Part model, mm, in its own coordinate system. A direction names the side the tool comes from. Coordinates: 2 decimals unless noted, no trailing zeros. Order: outer loops, then holes, each group sorted by start corner. A loop starts at its lowest first (then second) coordinate and runs counter-clockwise, first axis right, second up.
1) Cut at D-D (y = 27.5). List the corners of the cut face in (x, z), and give its area (3 significant figures).
2) Cut at C-C (x = -14). List the corners of the cut face in (y, z), and give its area (3 significant figures).
3) Pin check, flat tips, straight feed: pin 1 Ø0.9 at (x, y) = (-23.5, 33) entering from +Z; pin 2 Ø12 at (x, y) = (-24, -6.5) entering from -Z; pin 3 Ø1.2 at (x, z) = (-30.7, 5) entering from -Y; pin 4 Ø6 at (x, y) = (-41.5, 27) entering from +Z. Stop position of each tip, or through.
4) Cut at B-B (y = 2.5). List the corners of the cut face in (x, z), and give its area (3 significant figures).
5) Tool access for faces 1 (the cylindrical face through (-11.004, 31.9, 4.958)), 2 (the cylindrical face through (-31.7, -14.1, 5.1)), 3 (the flat face through (-18, 10.185, 1)), 4 (the flat face through (-10.704, 10, 5)): list every direction of +Z, -Z, +X, -X, +Y, -Y with a clear straight run to the whole face (end or side of a thin tool).
6) Wall check: L1, parallel to X at y = 32.5, z = 5; L2, parallel to Y at x = -36, z = 7; L3, parallel to Y at x = -33, z = 1.5. Give the ranges that are in metal, low to high.
7) Mould opens along Z. For faces 5 (the cylindrical face through (-43.7, -14.1, 5.1)), 6 (the flat face through (-28, -15, 8)), 7 (the cylindrical face through (-11.004, -13.53, 5.042)) say: +Z half, -Z half, draft (parallel to the pull), parting line (faces both ways), or undercut.
8) Cut at A-A (z = 5). Give the number of separate pieces and of enclosed holes in the cut face, and give its area (3 significant figures).
Autodesk Inventor part; units mm, degrees
ref_plane "YZ Plane" through (0, 0, 0) normal (1, 0, 0) x (0, 1, 0)
ref_plane "XZ Plane" through (0, 0, 0) normal (0, 1, 0) x (-1, 0, 0)
ref_plane "XY Plane" through (0, 0, 0) normal (0, 0, 1) x (1, 0, 0)
sketch "Sketch1" plane through (0, 0, 0) normal (0, 0, 1) x (1, 0, 0)
  line L0 (-45.7037, 34.1852) -> (-8.7037, 34.1852)
  line L1 (-8.7037, 34.1852) -> (-8.7037, -15.8148)
  line L2 (-8.7037, -15.8148) -> (-45.7037, -15.8148)
  line L3 (-45.7037, -15.8148) -> (-45.7037, 34.1852)
  line L4 (-43.7037, 32.1852) -> (-10.7037, 32.1852)
  line L5 (-10.7037, 32.1852) -> (-10.7037, -13.8148)
  line L6 (-10.7037, -13.8148) -> (-43.7037, -13.8148)
  line L7 (-43.7037, -13.8148) -> (-43.7037, 32.1852)
  point P0 (0, 0)
  dimension "d0" = 2
  dimension "d1" = 2
  dimension "d2" = 2
  dimension "d3" = 2
  dimension "d4" = 37
  dimension "d5" = 50
extrude "Extrusion1" add sketch "Sketch1" along normal blind 2
sketch "Sketch2" plane through (0, 0, 2) normal (0, 0, 1) x (1, 0, 0)
  line L0 (-43.7037, 32.1852) -> (-10.7037, 32.1852)
  line L1 (-10.7037, -13.8148) -> (-43.7037, -13.8148)
  line L2 (-43.7037, 32.1852) -> (-10.7037, -13.8148) construction
  line L3 (-44.5162, 31.6023) -> (-11.5162, -14.3977)
  line L4 (-9.8912, -13.2319) -> (-42.8912, 32.7681)
  arc A0 (-42.8912, 32.7681) -> (-44.5162, 31.6023) centre (-43.7037, 32.1852) ccw
  arc A1 (-11.5162, -14.3977) -> (-9.8912, -13.2319) centre (-10.7037, -13.8148) ccw
  line L5 (-10.7037, 32.1852) -> (-10.7037, -13.8148)
  line L6 (-10.7037, 32.1852) -> (-43.7037, -13.8148) construction
  line L7 (-11.5162, 32.7681) -> (-44.5162, -13.2319)
  line L8 (-42.8912, -14.3977) -> (-9.8912, 31.6023)
  arc A2 (-9.8912, 31.6023) -> (-11.5162, 32.7681) centre (-10.7037, 32.1852) ccw
  arc A3 (-44.5162, -13.2319) -> (-42.8912, -14.3977) centre (-43.7037, -13.8148) ccw
  point P0 (0, 0)
  point P1 (-27.2037, 9.1852)
  point P2 (-27.2037, 9.1852)
  point P3 (-25.973, 9.1852)
  point P4 (-27.2037, 10.9007)
  point P5 (-28.4344, 9.1852)
  point P6 (-27.2037, 7.4696)
  dimension "d8" = 2
  dimension "d9" = 2
extrude "Extrusion2" add sketch "Sketch2" against normal blind 2 contours L4 L7 L3 A0 | L7 A2 L8 L5 L0 | L0 L5 L8 L4 L7 | L4 L8 L3 L7 | L4 L5 L1 L3 L8 | L3 L8 A3 L7 | L4 A1 L3 L1 L5
sketch "Sketch3" plane through (0, 0, 2) normal (0, 0, 1) x (1, 0, 0)
  line L0 (-45.7037, 34.1852) -> (-45.7037, -15.8148)
  line L1 (-8.7037, -15.8148) -> (-8.7037, 34.1852)
  line L2 (-45.7037, 34.1852) -> (-8.7037, 34.1852)
  line L3 (-8.7037, 34.1852) -> (-8.7037, 32.1852)
  line L4 (-8.7037, 32.1852) -> (-45.7037, 32.1852)
  line L5 (-45.7037, 32.1852) -> (-45.7037, 34.1852)
  line L6 (-45.7037, -15.8148) -> (-8.7037, -15.8148)
  line L7 (-8.7037, -15.8148) -> (-8.7037, -13.8148)
  line L8 (-8.7037, -13.8148) -> (-45.7037, -13.8148)
  line L9 (-45.7037, -13.8148) -> (-45.7037, -15.8148)
  line L10 (-42.473, 32.1852) -> (-11.9344, 32.1852)
  line L11 (-11.9344, -13.8148) -> (-42.473, -13.8148)
  line L12 (-45.7037, -15.8148) -> (-8.7037, -15.8148)
  point P0 (0, 0)
  point P1 (-8.7037, 34.1852)
extrude "Extrusion3" add sketch "Sketch3" along normal blind 6 contours L2 L1 L4 L0 | L8 L1 L6 L0
sketch "Sketch4" plane through (-45.7037, 34.1852, 0) normal (0, 1, 0) x (1, 0, 0)
  line L0 (37, -8) -> (0, -8)
  line L1 (0, 0) -> (0, -8)
  point P0 (45.7037, 0)
  point P1 (3, -5)
  point P2 (15, -5)
  dimension "d14" = 3
  dimension "d15" = 3
  dimension "d16" = 3
  dimension "d17" = 12
hole "Hole1" at (-42.7037, 34.1852, 5) at (-30.7037, 34.1852, 5) direction (0, -1, 0) diameter 2 depth 10 tip angle 118 countersink diameter 5 countersink angle 90
sketch "Sketch5" plane through (-45.7037, -15.8148, 0) normal (0, -1, 0) x (1, 0, 0)
  circle A0 centre (15, 5) radius 1
  circle A1 centre (3, 5) radius 1
  point P0 (45.7037, 0)
hole "Hole2" at (-30.7037, -15.8148, 5) at (-42.7037, -15.8148, 5) direction (0, 1, 0) diameter 2 depth 10 tip angle 118 countersink diameter 5 countersink angle 90
sketch "Sketch6" plane through (0, 0, 0) normal (0, 0, -1) x (-1, 0, 0)
  line L0 (11.9344, -13.8148) -> (42.473, -13.8148)
  line L1 (43.7037, -12.0993) -> (43.7037, 30.4696)
  line L2 (17.7037, -13.8148) -> (43.7037, -13.8148)
  line L3 (43.7037, -13.8148) -> (43.7037, -6.8148)
  line L4 (43.7037, -6.8148) -> (17.7037, -6.8148)
  line L5 (17.7037, -6.8148) -> (17.7037, -13.8148)
  line L6 (17.7037, 32.1852) -> (43.7037, 32.1852)
  line L7 (43.7037, 32.1852) -> (43.7037, 25.1852)
  line L8 (43.7037, 25.1852) -> (17.7037, 25.1852)
  line L9 (17.7037, 25.1852) -> (17.7037, 32.1852)
  line L10 (42.473, 32.1852) -> (11.9344, 32.1852)
  line L11 (45.7037, 34.1852) -> (45.7037, -15.8148)
  line L12 (8.7037, 34.1852) -> (45.7037, 34.1852)
  line L13 (45.7037, -15.8148) -> (8.7037, -15.8148)
  point P0 (0, 0)
  dimension "d35" = 28
  dimension "d36" = 28
  dimension "d37" = 9
  dimension "d38" = 9
extrude "Extrusion4" cut sketch "Sketch6" against normal blind 2
sketch "Sketch7" plane through (0, 0, 0) normal (0, 0, -1) x (-1, 0, 0)
  line L0 (39.9127, -6.8148) -> (37.4513, -6.8148)
  line L1 (43.7037, -13.8148) -> (43.7037, 32.1852)
  line L2 (37.4513, -6.8148) -> (43.7037, -6.8148)
  line L3 (43.7037, -6.8148) -> (43.7037, -4.8148)
  line L4 (43.7037, -4.8148) -> (37.4513, -4.8148)
  line L5 (37.4513, -4.8148) -> (37.4513, -6.8148)
  line L6 (37.4513, 25.1852) -> (39.9127, 25.1852)
  line L7 (37.4513, 25.1852) -> (43.7037, 25.1852)
  line L8 (43.7037, 25.1852) -> (43.7037, 23.1852)
  line L9 (43.7037, 23.1852) -> (37.4513, 23.1852)
  line L10 (37.4513, 23.1852) -> (37.4513, 25.1852)
  point P0 (0, 0)
  dimension "d41" = 2
  dimension "d42" = 2
extrude "Extrusion5" add sketch "Sketch7" against normal blind 2
sketch "Sketch8" plane through (0, 0, 0) normal (0, 0, -1) x (-1, 0, 0)
  line L0 (10.7037, -12.0993) -> (25.973, 9.1852)
  line L1 (25.973, 9.1852) -> (10.7037, 9.1852) construction
  line L2 (10.7037, 30.4696) -> (10.7037, -12.0993)
  line L3 (25.973, 10.1852) -> (10.7037, 10.1852)
  line L4 (10.7037, 8.1852) -> (25.973, 8.1852)
  arc A0 (25.973, 8.1852) -> (25.973, 10.1852) centre (25.973, 9.1852) ccw
  arc A1 (10.7037, 10.1852) -> (10.7037, 8.1852) centre (10.7037, 9.1852) ccw
  point P0 (0, 0)
  point P1 (18.3383, 9.1852)
  dimension "d45" = 2
extrude "Extrusion6" add sketch "Sketch8" against normal blind 2 contours L4 L2 L3 A0 | A1 L2
sketch "Sketch9" plane through (-8.7037, -15.8148, 0) normal (1, 0, 0) x (0, 0, -1)
  line L0 (0, 50) -> (-8, 50)
  line L1 (0, 0) -> (-8, 0)
  line L2 (0, 50) -> (-10, 50)
  line L3 (-10, 50) -> (-10, 0)
  line L4 (-10, 0) -> (0, 0)
  line L5 (0, 0) -> (0, 50)
  point P0 (0, 15.8148)
  dimension "d48" = 10
extrude "Extrusion7" add sketch "Sketch9" against normal blind 2
fillet "Fillet1" radius 1 2 edges at (-10.7037, 32.1852, 5) (-10.7037, -13.8148, 5)
properties part number "face-1"
Geometry check:
1. outline: (-45.7, 0) - (-43.7, 0) - (-43.7, 2) - (-45.7, 2) - close; (-15.3, 0) - (-12.83, 0) - (-12.83, 2) - (-15.3, 2) - close; (-10.7, 0) - (-8.7, 0) - (-8.7, 10) - (-10.7, 10) - close
1. area: 28.9 mm2
2. outline: (-15.81, 0) - (-13.81, 0) - (-13.81, 8) - (-15.81, 8) - close; (-10.94, 0) - (-7.5, 0) - (-7.5, 2) - (-10.94, 2) - close; (8.19, 0) - (10.19, 0) - (10.19, 2) - (8.19, 2) - close; (25.87, 0) - (29.31, 0) - (29.31, 2) - (25.87, 2) - close; (32.19, 0) - (34.19, 0) - (34.19, 8) - (32.19, 8) - close
2. area: 49.7 mm2
3. pin 1: stops at z = 8
3. pin 2: stops at z = 0
3. pin 3: passes through
3. pin 4: stops at z = 2
4. outline: (-45.7, 0) - (-43.7, 0) - (-43.7, 2) - (-45.7, 2) - close; (-33.23, 0) - (-30.77, 0) - (-30.77, 2) - (-33.23, 2) - close; (-23.64, 0) - (-21.18, 0) - (-21.18, 2) - (-23.64, 2) - close; (-10.7, 0) - (-8.7, 0) - (-8.7, 10) - (-10.7, 10) - close
4. area: 33.8 mm2
5. face 1: +Z, -X
5. face 2: +Y, -Y
5. face 3: +Z, -Z
5. face 4: +Z
6. L1: x = -45.7 to -43.7, -41.7 to -31.7, -29.7 to -8.7
6. L2: y = -15.81 to -13.81, 32.19 to 34.19
6. L3: y = -15.81 to -13.81, -0.61 to 2.82, 15.55 to 18.98, 32.19 to 34.19
7. face 5: undercut
7. face 6: +Z half
7. face 7: draft
8. separate pieces: 5
8. enclosed holes: 0
8. area: 215 mm2
